The model under review builds one solid part; all positions refer to its coordinate system, in mm. A direction names the side the tool comes from. Coordinates: 2 decimals unless noted, no trailing zeros. Loops run counter-clockwise (first coordinate to the right, second up) from the corner with the lowest first, then second, coordinate; pieces in that order, holes last. Notation, with made-up numbers: M 64.25,6.25 L 81.25,6.25 A21 ccw 81.25,36.25 Z; hole C 75,-6.5 d6. An arc over 180 degrees is marked long. Use one line per item in the form item = value.
```python
from build123d import *

# Parameters (mm, degrees)
F0_R          = 45.72
F1_DEPTH      = 8.89
F2_R          = 28.575
F3_DEPTH      = 63.5
F5_DEPTH      = 45.721
F5_DEPTH_BACK = 45.721
F6_R          = 45.72
F7_DEPTH      = 8.89
F8_R          = 7.62
F9_DEPTH      = 86.13506459
F10_R         = 2.2225
F11_DEPTH     = 8.89
F12_R         = 2.2225
F13_DEPTH     = 8.89


with BuildPart() as f1:
    # F0 (on Top) → F1 (new body)
    with BuildSketch(Plane.XY):
        Circle(F0_R)
    extrude(amount=F1_DEPTH)

    # F2 (on face) → F3 (join)
    with BuildSketch(Plane.XY.offset(8.89)):
        Circle(F2_R)
    extrude(amount=F3_DEPTH)

    # F4 (on Front) → F5 (cut, two sides)
    with BuildSketch(Plane.XZ) as f5_sk:
        Polygon((28.575, 72.39), (-28.575, 72.39), (28.575, 50.165), align=None)
    extrude(amount=-F5_DEPTH, mode=Mode.SUBTRACT)
    extrude(f5_sk.sketch, amount=F5_DEPTH_BACK, mode=Mode.SUBTRACT)

    # F6 (on face) → F7 (join)
    with BuildSketch(Plane(origin=(20.6996380697, 0, 53.2276407507), x_dir=(0.9320046715, 0, -0.3624462612), z_dir=(0.3624462612, 0, 0.9320046715))):
        with Locations((-22.2098007679, 0)):
            Circle(F6_R)
    extrude(amount=F7_DEPTH)

    # F8 (on face) → F9 (cut, through all)
    with BuildSketch(Plane(origin=(0, 0, 0), x_dir=(1, 0, 0), z_dir=(0, 0, -1))):
        Circle(F8_R)
    extrude(amount=-F9_DEPTH, mode=Mode.SUBTRACT)

    # F10 (on face) → F11 (cut, through all)
    with BuildSketch(Plane(origin=(0, 0, 0), x_dir=(1, 0, 0), z_dir=(0, 0, -1))):
        with Locations((0, -38.1)):
            Circle(F10_R)
        with Locations((38.1, 0)):
            Circle(F10_R)
        with Locations((0, 38.1)):
            Circle(F10_R)
        with Locations((-38.1, 0)):
            Circle(F10_R)
    extrude(amount=-F11_DEPTH, mode=Mode.SUBTRACT)

    # F12 (on face) → F13 (cut, through all)
    with BuildSketch(Plane(origin=(23.9217853314, 0, 61.5131622807), x_dir=(0.9320046715, 0, -0.3624462612), z_dir=(0.3624462612, 0, 0.9320046715))):
        with Locations((-22.2098007679, -38.1)):
            Circle(F12_R)
        with Locations((15.8901992321, 0)):
            Circle(F12_R)
        with Locations((-60.3098007679, 0)):
            Circle(F12_R)
        with Locations((-22.2098007679, 38.1)):
            Circle(F12_R)
    extrude(amount=-F13_DEPTH, mode=Mode.SUBTRACT)


solid = f1.part
```
1. Add section C-C (y = -38.1). State the section outline as (x, z) points, then the cut area to 3 significant figures.
Response values:
outline = M -25.27,0 L -2.22,0 L -2.22,8.89 L -25.27,8.89 Z; M -23.55,70.44 L -2.07,62.08 L 1.15,70.37 L -20.33,78.72 Z; M 2.07,60.47 L 23.55,52.12 L 26.78,60.4 L 5.29,68.76 Z; M 2.22,0 L 25.27,0 L 25.27,8.89 L 2.22,8.89 Z
area = 820 mm^2
2. Add section D-D (y = 17). State the section outline as (x, z) points, then the cut area to 3 significant figures.
Response values:
outline = M -42.44,0 L 42.44,0 L 42.44,8.89 L 22.97,8.89 L 22.97,52.35 L 39.56,45.89 L 42.78,54.18 L -36.33,84.95 L -39.56,76.66 L -22.97,70.21 L -22.97,8.89 L -42.44,8.89 Z
area = 3,920 mm^2
3. Insertion check: P1, Ø6, axis at x = 38.1, y = 0, coming from the +Z side; P2, Ø6, axis at y = 28, z = 30, coming from the -X side; P3, Ø3, axis at x = 11.5, z = 43, coming from the +Y side; P4, Ø17.5, axis at x = 0, y = 0, coming from the -Z side. Each pin has a flat end and moves straight along its axis. Give the tip position at first contact, or say it passes through.
Response values:
P1 = 57.17
P2 = -13.84
P3 = 26.77
P4 = 0
4. The part is to be moulded in two halves that separate along Y. For faces 1 (the face through (-28.547, 1.256, 33.14)), 2 (the face through (-21, -20, 8.89)), 3 (the face through (-36.047, 0.851, 4.383)), say which applies: pulls with the +Y half, pulls with the -Y half, needs draft (parallel to the pull), parting line crosses it, or undercut.
Response values:
face_1 = parting line crosses it
face_2 = needs draft
face_3 = undercut
5. Add section A-A (y = -3.5). State the section outline as (x, z) points.
Response values:
outline = M -45.59,0 L -6.77,0 L -6.77,73.45 L -39.26,86.09 L -42.49,77.8 L -28.36,72.31 L -28.36,8.89 L -45.59,8.89 Z; M 6.77,0 L 45.59,0 L 45.59,8.89 L 28.36,8.89 L 28.36,50.25 L 42.49,44.76 L 45.71,53.04 L 6.77,68.18 Z
6. Machinability: for faces 4 (the face through (-0.6, -29.84, 61.51)), 5 (the face through (40.153, 0.851, 4.383)), 6 (the face through (-6.047, 4.637, 36.434)), which of the approach directions +Z, -Z, +X, -X, +Y, -Y give a long, thin tool a straight path to every point of the face, cutting with its end or side? Answer none if there is none.
Response values:
face_4 = none
face_5 = -Z
face_6 = +Z, -Z
7. Wall thickness on line 1 along Y through (x, z) = (0, 6.25); line 2 along X through (y, z) = (0.5, 33); line 3 along X through (y, z) = (0, 47) (3 decimals): over which ranges is each line inside the solid? List them lowest first. Write a range as from..to.
Response values:
line_1 = -45.72..-40.32, -35.88..-7.62, 7.62..35.88, 40.32..45.72
line_2 = -28.57..-7.6, 7.6..28.57
line_3 = -28.575..-7.62, 7.62..28.575, 37.712..43.503
8. Add section B-B (z = 41.5). State the section outline as (x, y) points (3 decimals), then the cut area to 3 significant figures.
Response values:
outline = C 0,0 d57.15; hole C 0,0 d15.24
area = 2,380 mm^2
